Design review of the part built by this model. Coordinates are the model's own, in mm. A direction names the side the tool comes from. Round coordinates to 2 decimals unless told otherwise and drop trailing zeros. Loops run counter-clockwise (first coordinate to the right, second up) from the corner with the lowest first, then second, coordinate; pieces in that order, holes last. Notation, with made-up numbers: M 72.25,-38 L 121.25,-38 A6 ccw 121.25,-31 Z; hole C 16,46.5 d3. An arc over 180 degrees is marked long. One line per item, written item: value. Start each with the question number.
Item 1: For faces 1 (the flat face through (-6, 138, 0)), 2 (the flat face through (-7, 280, 0)), list the 3-axis set-ups (+Z, -Z, +X, -X, +Y, -Y) from which the entire face can be reached by the end or side of a thin tool; tool diameter is ignored.
Item 2: Mouldability with a two-part tool opening along Z and no side actions: class faces 3 (the flat face through (0, 138, -6)), 4 (the flat face through (-7, 0, 0)), 5 (the flat face through (0, 138, -7.5)), 6 (the flat face through (0, 138, 7.5)) as released by +Z, released by -Z, zero draft, split by the parting line, or undercut.
Item 3: For line 1 along Y through (x, z) = (0, -6.9); line 2 along Y through (x, z) = (-7.15, 0); line 3 along X through (y, z) = (182.5, 6.7), list the stretches that pass through material, from the lowest coordinate up.
Item 4: Clearance check with flat-ended pins moving along their axes: pin 1 (3 mm diameter, centred on x = 0, y = 47.5, fed in from -Z); pin 2 (4.5 mm diameter, centred on y = 247.5, z = 0, fed in from -X). State where each tip first meets the part, or that it passes through.
Item 5: We need section A-A (y = 74). Write out the cut boundary in (x, z), then the cut area to 3 significant figures.
from build123d import *

# Parameters (mm, degrees)
SKETCH_1_W          = 15
SKETCH_1_H          = 15
SKETCH_1_W_2        = 12
SKETCH_1_H_2        = 12
EXTRUDE_1_DEPTH     = 280
SKETCH_2_R          = 2
CUT_EXTRUDE_1_DEPTH = 281.501782526
SKETCH_3_R          = 2
CUT_EXTRUDE_2_DEPTH = 281.501782526


with BuildPart() as part:
    # ｽｹｯﾁ1 → 押し出し-薄板1 (new body)
    with BuildSketch(Plane(origin=(0, 0, 0), x_dir=(1, 0, 0), z_dir=(0, 1, 0))):
        Rectangle(SKETCH_1_W, SKETCH_1_H)
        Rectangle(SKETCH_1_W_2, SKETCH_1_H_2, mode=Mode.SUBTRACT)
    extrude(amount=EXTRUDE_1_DEPTH)

    # ｽｹｯﾁ2 → ｶｯﾄ - 押し出し1 (cut, through all)
    with BuildSketch(Plane(origin=(7.5, 0, 0), x_dir=(0, 0, -1), z_dir=(1, 0, 0))):
        with Locations((0, 272.5)):
            Circle(SKETCH_2_R)
        with Locations((0, 247.5)):
            Circle(SKETCH_2_R)
    extrude(amount=-CUT_EXTRUDE_1_DEPTH, mode=Mode.SUBTRACT)

    # ｽｹｯﾁ3 → ｶｯﾄ - 押し出し2 (cut, through all)
    with BuildSketch(Plane.XY.offset(7.5)):
        with Locations((0, 7.5)):
            Circle(SKETCH_3_R)
        with Locations((0, 47.5)):
            Circle(SKETCH_3_R)
        with Locations((0, 182.5)):
            Circle(SKETCH_3_R)
    extrude(amount=-CUT_EXTRUDE_2_DEPTH, mode=Mode.SUBTRACT)


solid = part.part
A:
1. face 1: +Y, -Y
1. face 2: +Z, -Z, +X, -X, +Y
2. face 3: undercut
2. face 4: zero draft
2. face 5: released by -Z
2. face 6: released by +Z
3. line 1: 0 to 5.5, 9.5 to 45.5, 49.5 to 180.5, 184.5 to 280
3. line 2: 0 to 245.5, 249.5 to 270.5, 274.5 to 280
3. line 3: -7.5 to -2, 2 to 7.5
4. pin 1: through
4. pin 2: x = -7.5
5. outline: M -7.5,-7.5 L 7.5,-7.5 L 7.5,7.5 L -7.5,7.5 Z; hole M -6,-6 L 6,-6 L 6,6 L -6,6 Z
5. area: 81.0 mm2
